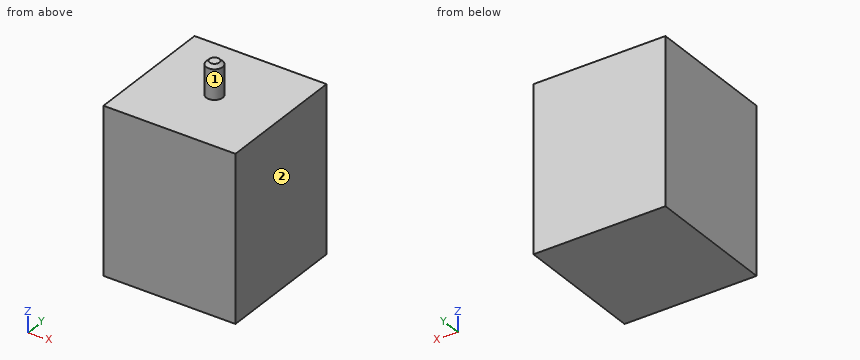
from build123d import *

# Parameters (mm, degrees)
F0_W     = 80
F0_H     = 80
F1_DEPTH = 100
F2_R     = 5
F3_DEPTH = 20
F4_SIZE  = 2


with BuildPart() as f1:
    # F0 (on Top) → F1 (new body)
    with BuildSketch(Plane.XY):
        with Locations((0.311533, 2.066482)):
            Rectangle(F0_W, F0_H)
    extrude(amount=F1_DEPTH)

    # F2 (on face) → F3 (join)
    with BuildSketch(Plane.XY.offset(100)):
        with Locations((0, 2.066482)):
            Circle(F2_R)
    extrude(amount=F3_DEPTH)

    # F4
    f4_edges = [f1.edges().sort_by_distance(p)[0] for p in [
        (-5, 2.066482, 120),
    ]]
    chamfer(f4_edges, length=F4_SIZE)


solid = f1.part
The listing builds one solid part. Answer for the finished solid, in the listing's coordinates (mm). Face numbers are marked on the shaded views. A direction names the side the tool comes from. Round coordinates to 2 decimals unless told otherwise and drop trailing zeros. Order: outer loops, then holes, each group sorted by start corner. A loop starts at its lowest first (then second) coordinate and runs counter-clockwise, first axis right, second up. Notation, with made-up numbers: (10.25, -13) -> (24.25, -13) arc R22 ccw to (24.25, -7) -> close; hole circle Ø1 at (44.25, 67.25). An arc over 180 degrees is marked (long way). Put each result on its own line as item: value.
Q1. Which of the six approach directions +Z, -Z, +X, -X, +Y, -Y give full straight-line access (tool end or side, diameter ignored) to the marked faces 1 and 2?
Results list:
face 1: +Z
face 2: +Z, -Z, +X, +Y, -Y
Q2. Section B-B, the plane y = -27 is taken. Write down the section's boundary in (x, z), and give its area (3 significant figures).
Results list:
outline: (-39.69, 0) -> (40.31, 0) -> (40.31, 100) -> (-39.69, 100) -> close
area: 8,000 mm^2
Q3. Section C-C, the plane z = 111 is taken. Write down the section's boundary in (x, y).
Results list:
outline: circle Ø10 at (0, 2.07)
Q4. Consider line 1 along Z through (x, y) = (26, -22.5). Determine where the line is inside the solid, lowest interval first.
Results list:
line 1: 0 to 100
Q5. Each of these flat-tipped pins is pushed along its axis until it touches: P1, Ø8, axis at x = 13.5, y = -15.5, coming from the +Z side; P2, Ø12, axis at x = -0.5, y = 13, coming from the +Z side. Where does it stop, or does it pass through?
Results list:
P1: z = 100
P2: z = 118.06
Q6. Section D-D, the plane x = -12 is taken. Write down the section's boundary in (y, z).
Results list:
outline: (-37.93, 0) -> (42.07, 0) -> (42.07, 100) -> (-37.93, 100) -> close
Q7. Section A-A, the plane x = 0 is taken. Write down the section's boundary in (y, z).
Results list:
outline: (-37.93, 0) -> (42.07, 0) -> (42.07, 100) -> (7.07, 100) -> (7.07, 118) -> (5.07, 120) -> (-0.93, 120) -> (-2.93, 118) -> (-2.93, 100) -> (-37.93, 100) -> close
